from build123d import *

# Parameters (mm, degrees)
SKETCH1_R           = 1.5
BOSS_EXTRUDE1_DEPTH = 1.5


with BuildPart() as part:
    # Sketch1 → Boss-Extrude1 (new body)
    with BuildSketch(Plane(origin=(0, 0, 0), x_dir=(1, 0, 0), z_dir=(0, 1, 0))):
        Polygon((-22.75, -50.75), (11.75, -50.75), (14.75, -47.75), (26.75, -47.75), (26.75, 50.75), (25.85, 50.75), (-20.75, 50.75), (-25.85, 50.75), (-26.75, 50.75), (-26.75, -47.75), (-25.75, -47.75), align=None)
        with Locations(Location((-24.35, -45.75, 0), (0, 0, 270))):
            Circle(SKETCH1_R, mode=Mode.SUBTRACT)
        with BuildLine():
            ThreePointArc((-17.75, -15.25), (-19.25, -16.75), (-20.75, -15.25))
            ThreePointArc((-20.75, -15.25), (-19.25, -13.75), (-17.75, -15.25))
        make_face(mode=Mode.SUBTRACT)
        with Locations(Location((24.35, -37.5, 0), (0, 0, 270))):
            Circle(SKETCH1_R, mode=Mode.SUBTRACT)
        with Locations(Location((8.75, -15.25, 0), (0, 0, 270))):
            Circle(SKETCH1_R, mode=Mode.SUBTRACT)
        with Locations(Location((-24.35, 38.25, 0), (0, 0, 270))):
            Circle(SKETCH1_R, mode=Mode.SUBTRACT)
        with BuildLine():
            ThreePointArc((24.35, 35.5), (23.289339828, 38.060660172), (25.85, 37))
            ThreePointArc((25.85, 37), (25.410660172, 35.939339828), (24.35, 35.5))
        make_face(mode=Mode.SUBTRACT)
    extrude(amount=BOSS_EXTRUDE1_DEPTH)


solid = part.part
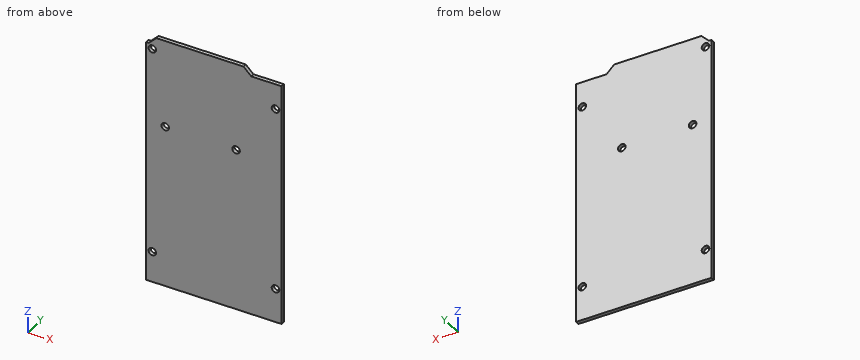
Check sheet for the modelled part. Datum: model origin and axes. Units: mm. Round coordinates to 2 decimals unless told otherwise and drop trailing zeros. Loops run counter-clockwise (first coordinate to the right, second up) from the corner with the lowest first, then second, coordinate; pieces in that order, holes last. Notation, with made-up numbers: M 84,-18.75 L 88,-18.75 A17 ccw 88,-12.75 Z; hole C 63.25,-19 d6. An arc over 180 degrees is marked long. One line per item, written item: value.
(1) Depth check by flat-ended pin: pin 1 Ø0.8 at (x, y) = (-26.5, 1) entering from +Z; pin 2 Ø2.5 at (x, z) = (-24.35, 45.75) entering from +Y. Enter the tip coordinate at first touch or a pass-through.
Computed values:
pin 1: stops at z = 47.75
pin 2: passes through
(2) Sectioned sample at A-A, the plane x = -24.35. Record the cut outline in (y, z), then the cut area to 3 significant figures.
Computed values:
outline: M 0,-50.75 L 1.5,-50.75 L 1.5,-39.75 L 0,-39.75 Z; M 0,-36.75 L 1.5,-36.75 L 1.5,44.25 L 0,44.25 Z; M 0,47.25 L 1.5,47.25 L 1.5,49.15 L 0,49.15 Z
area: 141 mm^2
(3) Sectioned sample at D-D, the plane z = 15.25. Record the cut outline in (x, y), then the cut area to 4 significant figures.
Computed values:
outline: M -26.75,0 L -20.75,0 L -20.75,1.5 L -26.75,1.5 Z; M -17.75,0 L 7.25,0 L 7.25,1.5 L -17.75,1.5 Z; M 10.25,0 L 26.75,0 L 26.75,1.5 L 10.25,1.5 Z
area: 71.25 mm^2
(4) Thickness scan on line 1 (X direction, y = 0.4, z = 15.25); line 2 (Z direction, x = -25, y = 0.5); line 3 (X direction, y = 1.25, z = 37.5). Record the ranges inside material, lowest first.
Computed values:
line 1: x = -26.75 to -20.75, -17.75 to 7.25, 10.25 to 26.75
line 2: z = -50.75 to -39.6, -36.9 to 44.4, 47.1 to 48.5
line 3: x = -26.75 to 22.85, 25.85 to 26.75
(5) Sectioned sample at B-B, the plane y = 0.45. Record the cut outline in (x, z).
Computed values:
outline: M -26.75,-50.75 L 26.75,-50.75 L 26.75,47.75 L 14.75,47.75 L 11.75,50.75 L -22.75,50.75 L -25.75,47.75 L -26.75,47.75 Z; hole C -24.35,-38.25 d3; hole C -24.35,45.75 d3; hole C -19.25,15.25 d3; hole C 8.75,15.25 d3; hole C 24.35,-37 d3; hole C 24.35,37.5 d3
(6) Sectioned sample at C-C, the plane x = 8.75. Record the cut outline in (y, z).
Computed values:
outline: M 0,-50.75 L 1.5,-50.75 L 1.5,13.75 L 0,13.75 Z; M 0,16.75 L 1.5,16.75 L 1.5,50.75 L 0,50.75 Z
